Build history of the part. All positions in model axes, mm. A direction names the side the tool comes from. Coordinates: 2 decimals unless noted, no trailing zeros. Order: outer loops, then holes, each group sorted by start corner. A loop starts at its lowest first (then second) coordinate and runs counter-clockwise, first axis right, second up. Notation, with made-up numbers: (36, 20) - (75, 20) arc R16 cw to (75, 31) - close; hole circle Ø2 at (47.25, 57). An arc over 180 degrees is marked (long way). Return JSON: item names as keys, results as strings.
from build123d import *

# Parameters (mm, degrees)
SKETCH_1_R          = 40
EXTRUDE_1_DEPTH     = 3
SKETCH_2_R          = 27
EXTRUDE_2_DEPTH     = 5
SKETCH_3_R          = 3
CUT_EXTRUDE_1_DEPTH = 5


with BuildPart() as part:
    # 草图1 → 凸台-拉伸1 (new body)
    with BuildSketch(Plane.XY):
        Circle(SKETCH_1_R)
    extrude(amount=EXTRUDE_1_DEPTH)

    # 草图2 → 凸台-拉伸2 (add)
    with BuildSketch(Plane.XY.offset(3)):
        Circle(SKETCH_2_R)
    extrude(amount=EXTRUDE_2_DEPTH)

    # 草图3 → 切除-拉伸1 (cut)
    with BuildSketch(Plane(origin=(0, 0, 0), x_dir=(-1, 0, 0), z_dir=(0, 0, -1))):
        with Locations((35, 0)):
            Circle(SKETCH_3_R)
        with Locations((-35, 0)):
            Circle(SKETCH_3_R)
    extrude(amount=-CUT_EXTRUDE_1_DEPTH, mode=Mode.SUBTRACT)


solid = part.part
1. Cut at B-B on x = 34. Give the cut face in (y, z), plus the area to 3 significant figures.
Check values:
{"outline": "(-21.07, 0) - (-2.83, 0) - (-2.83, 3) - (-21.07, 3) - close; (2.83, 0) - (21.07, 0) - (21.07, 3) - (2.83, 3) - close", "area": "109 mm²"}
2. Tool access for faces 1 (the flat face through (8, -26, 3)), 2 (the flat face through (0, 0, 8)): list every direction of +Z, -Z, +X, -X, +Y, -Y with a clear straight run to the whole face (end or side of a thin tool).
Check values:
{"face 1": "+Z", "face 2": "+Z, +X, -X, +Y, -Y"}
3. Mould opens along X. For faces 3 (the cylindrical face through (38, 0, 1)), 4 (the cylindrical face through (-5.85, -26.36, 5.46)), 5 (the flat face through (-1, 1, 0)) say: pulls with the +X half, pulls with the -X half, needs draft (parallel to the pull), parting line crosses it, or undercut.
Check values:
{"face 3": "undercut", "face 4": "parting line crosses it", "face 5": "needs draft"}
4. Cut at C-C on z = 1.75. Give the cut face in (x, y), plus the area to 3 significant figures.
Check values:
{"outline": "circle Ø80 at (0, 0); hole circle Ø6 at (-35, 0); hole circle Ø6 at (35, 0)", "area": "4,970 mm²"}
5. Cut at A-A on y = 0. Give the cut face in (x, z).
Check values:
{"outline": "(-40, 0) - (-38, 0) - (-38, 3) - (-40, 3) - close; (-32, 0) - (32, 0) - (32, 3) - (27, 3) - (27, 8) - (-27, 8) - (-27, 3) - (-32, 3) - close; (38, 0) - (40, 0) - (40, 3) - (38, 3) - close"}
6. Drop flat-ended pins along their axis: pin 1 (1 mm diameter, centred on y = 3.5, z = 4, fed in from +X); pin 2 (9.5 mm diameter, centred on x = 35, y = 0, fed in from +Z); pin 3 (1 mm diameter, centred on y = 29.5, z = 2, fed in from -X). Give the stop position or say it passes through.
Check values:
{"pin 1": "x = 26.83", "pin 2": "z = 3", "pin 3": "x = -27.55"}
7. Cut at D-D on x = 0. Give the cut face in (y, z), plus the area to 3 significant figures.
Check values:
{"outline": "(-40, 0) - (40, 0) - (40, 3) - (27, 3) - (27, 8) - (-27, 8) - (-27, 3) - (-40, 3) - close", "area": "510 mm²"}
8. Probe L1, parallel to Z at x = 29, y = 6; L2, parallel to Y at x = -35, z = 1; L3, parallel to Y at x = -19.5, z = 2.5. List the from-to ranges inside material, lowest first.
Check values:
{"L1": "0 to 3", "L2": "-19.36 to -3, 3 to 19.36", "L3": "-34.92 to 34.92"}
